Autodesk Inventor part; units mm, degrees
ref_plane "РабПлоскость1" through (25, 2, 0) normal (1, 0, 0) x (0, 0, -1)
ref_plane "РабПлоскость2" through (2, 12.5, 0) normal (0, -1, 0) x (1, 0, 0)
ref_plane "РабПлоскость3" through (25, 25, 5.2) normal (1, 0, 0) x (0, 0, -1)
sketch "Эскиз1" plane through (0, 0, 0) normal (0, 0, 1) x (1, 0, 0)
  line L0 (0, 0) -> (50, 0)
  line L1 (50, 0) -> (50, 25)
  line L2 (50, 25) -> (0, 25)
  line L3 (0, 25) -> (0, 0)
  dimension "d0" = 50
  dimension "d1" = 25
extrude "Выдавливание1" add sketch "Эскиз1" along normal blind 5.2
shell "Оболочка1" thickness 2 removed faces 1 at (16.6667, 16.6667, 0)
sketch "Эскиз2" plane through (0, 0, 5.2) normal (0, 0, 1) x (1, 0, 0)
  line L0 (50, 25) -> (0, 25)
  line L1 (25, 25) -> (25, 0)
  line L2 (0, 0) -> (50, 0)
  line L3 (25, 12.5) -> (12, 12.5)
  line L4 (0, 25) -> (0, 0)
  circle A0 centre (12, 12.5) radius 8.1
  circle A1 centre (38, 12.5) radius 8.1
  line L5 (25, 25) -> (25, 20)
  line L6 (21.75, 20) -> (28.25, 20) construction
  line L7 (21.75, 18) -> (28.25, 18)
  line L8 (28.25, 22) -> (21.75, 22)
  arc A2 (21.75, 22) -> (21.75, 18) centre (21.75, 20) ccw
  arc A3 (28.25, 18) -> (28.25, 22) centre (28.25, 20) ccw
  point P0 (25, 18)
  point P1 (25, 22)
  dimension "d5" = 13
  dimension "d6" = 16.2
  dimension "d9" = 5
  dimension "d10" = 3.25
  dimension "d11" = 4
extrude "Выдавливание2" cut sketch "Эскиз2" against normal through all contours L8 A3 L7 L1 | L1 L7 A2 L8 | A0 | A1
sketch "Эскиз5" plane through (48, 23, 3.2) normal (0, 0, -1) x (-1, 0, 0)
  line L0 (0, 0) -> (1.05, 0)
  line L1 (0, 0) -> (46, 0)
  line L2 (1.05, 0) -> (1.05, -1.05)
  circle A0 centre (1.05, -1.05) radius 1.05
  line L3 (2.1, -2.1) -> (0, -2.1)
  line L4 (0, -2.1) -> (0, 0)
  line L5 (0, 0) -> (2.1, 0)
  line L6 (2.1, 0) -> (2.1, -2.1)
  line L7 (2.1, -2.1) -> (0, 0) construction
  line L8 (0, -2.1) -> (2.1, 0) construction
  point P0 (48, -23)
  point P1 (1.05, -2.1)
  point P2 (2.1, -1.05)
  dimension "d17" = 1.05
  dimension "d18" = 1.05
extrude "Выдавливание4" add sketch "Эскиз5" along normal blind 1 contours L0 A0 L4 | L1 L6 A0 | A0 | A0 L3 L4
ref_plane "РабПлоскость1" through (25, 2, 0) normal (1, 0, 0) x (0, 0, -1)
ref_plane "РабПлоскость2" through (2, 12.5, 0) normal (0, -1, 0) x (1, 0, 0)
mirror "Зеркальное отражение1" about plane through (2, 12.5, 0) normal (0, -1, 0) of "Выдавливание4"
mirror "Зеркальное отражение2" about plane through (25, 2, 0) normal (1, 0, 0) of "Выдавливание4", "Зеркальное отражение1"
sketch "Эскиз10" plane through (0, 0, 0) normal (0, -1, 0) x (1, 0, 0)
  line L0 (0, 0) -> (50, 0)
  line L1 (50, 0) -> (42, 0)
  line L2 (42, 0) -> (42, -8)
  line L3 (42, -8) -> (50, -8)
  line L4 (50, -8) -> (50, 0)
  dimension "d39" = 8
  dimension "d40" = 8
extrude "Выдавливание8" add sketch "Эскиз10" against normal up to surface (2 mm away)
sketch "Эскиз11" plane through (48, 2, 0) normal (0, 1, 0) x (1, 0, 0)
  line L0 (-6, 0) -> (-6, 8)
  line L1 (-6, 4) -> (2, 4)
  line L2 (2, 0) -> (2, 8)
  line L3 (-6, 8) -> (-6, 0)
  point P0 (-48, 0)
  point P1 (-2, 4)
hole "Отверстие2" at (46, 2, -4) direction (0, -1, 0) diameter 3.2 end through all countersink diameter 6 countersink angle 90
ref_plane "РабПлоскость3" through (25, 25, 5.2) normal (1, 0, 0) x (0, 0, -1)
mirror "Зеркальное отражение4" about plane through (25, 25, 5.2) normal (1, 0, 0) of "Отверстие2", "Выдавливание8"
fillet "Сопряжение2" radius 4 6 edges at (42, 1, -8) (50, 1, -8) (8, 1, -8) (0, 1, -8) (8, 1, 0) (42, 1, 0)
sketch "Эскиз12" plane through (0, 0, 5.2) normal (0, -1, 0) x (1, 0, 0)
  circle A0 centre (46, -9.2) radius 1.6
  circle A1 centre (4, -9.2) radius 1.6
  arc A2 (0, -9.2) -> (8, -9.2) centre (4, -9.2) ccw
  arc A3 (12, -5.2) -> (8, -9.2) centre (12, -9.2) ccw
  line L0 (12, -5.2) -> (38, -5.2)
  arc A4 (42, -9.2) -> (38, -5.2) centre (38, -9.2) ccw
  arc A5 (42, -9.2) -> (50, -9.2) centre (46, -9.2) ccw
  line L1 (50, -9.2) -> (50, 0)
  line L2 (0, 0) -> (50, 0)
  line L3 (0, -9.2) -> (0, 0)
  point P0 (0, -5.2)
extrude "Выдавливание9" add sketch "Эскиз12" along normal blind 1
properties part number "Крепление ультрасоника"
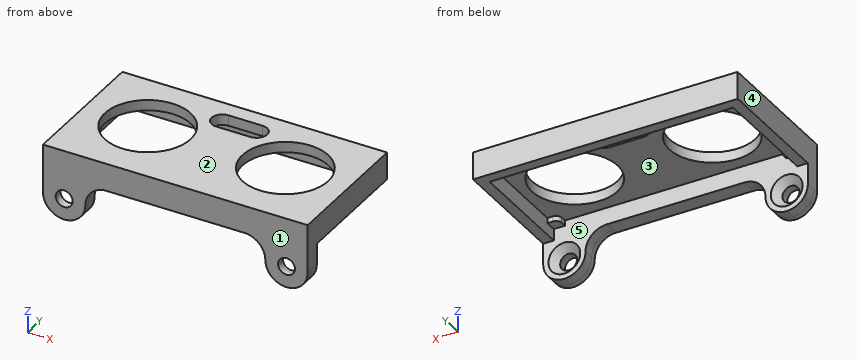
Can you work these out from the model? Positions are in its coordinate system, mm. Face numbers are marked on the shaded views. A direction names the side the tool comes from. Give positions to 0.01 mm unless a question says otherwise; leave off trailing zeros. Order: outer loops, then holes, each group sorted by start corner. A loop starts at its lowest first (then second) coordinate and runs counter-clockwise, first axis right, second up. Notation, with made-up numbers: M 25,-32.5 L 62,-32.5 A24 cw 62,-8.5 Z; hole C 22,-16.5 d11. An arc over 180 degrees is marked long. One line per item, written item: value.
Item 1: If we mould it in two halves opening along Y, with no side actions, what happens to the marked faces 1, 2 and 3? For each: pulls with the +Y half, pulls with the -Y half, needs draft (parallel to the pull), parting line crosses it, or undercut.
Verdict:
face 1: pulls with the -Y half
face 2: needs draft
face 3: undercut
Item 2: If we section it at D-D on y = 2.5: Write out the boundary of the cut face in (x, z).
Verdict:
outline: M 0,0 L 2,0 L 2,2.2 L 4.1,2.2 L 4.1,3.2 L 45.9,3.2 L 45.9,2.2 L 48,2.2 L 48,0 L 50,0 L 50,5.2 L 0,5.2 Z
Item 3: If we section it at B-B on x = 31: Write out the boundary of the cut face in (y, z).
Verdict:
outline: M -1,0 L 2,0 L 2,3.2 L 8.42,3.2 L 8.42,5.2 L -1,5.2 Z; M 16.58,3.2 L 23,3.2 L 23,0 L 25,0 L 25,5.2 L 16.58,5.2 Z
Item 4: If we section it at A-A on y = 12.5: Write out the boundary of the cut face in (x, z), and give its area (3 significant figures).
Verdict:
outline: M 0,0 L 2,0 L 2,3.2 L 3.9,3.2 L 3.9,5.2 L 0,5.2 Z; M 20.1,3.2 L 29.9,3.2 L 29.9,5.2 L 20.1,5.2 Z; M 46.1,3.2 L 48,3.2 L 48,0 L 50,0 L 50,5.2 L 46.1,5.2 Z
area: 48.0 mm2
Item 5: Please list where these lines run through material, in increasing order: line 1 (X direction, y = -0.3, z = -4); line 2 (Y direction, x = 38, z = 4.3); line 3 (Z direction, x = 46, y = 0.35).
Verdict:
line 1: 0 to 2.4, 5.6 to 8, 42 to 44.4, 47.6 to 50
line 2: -1 to 4.4, 20.6 to 25
line 3: -8 to -5.6, -2.4 to 5.2
Item 6: If we section it at C-C on z = 4.25: Write out the boundary of the cut face in (x, y).
Verdict:
outline: M 0,-1 L 50,-1 L 50,25 L 0,25 Z; hole C 12,12.5 d16.2; hole M 21.75,18 L 28.25,18 A2 ccw 28.25,22 L 21.75,22 A2 ccw Z; hole C 38,12.5 d16.2
Item 7: For the marked faces 4 and 5, which set-ups out of +Z, -Z, +X, -X, +Y, -Y let a thin tool reach every point of the face, with its end or its side?
Verdict:
face 4: +Z, -Z, -X, +Y, -Y
face 5: -Z
Item 8: For pin 1 (1 mm diameter, centred on x = 22.5, y = 18, fed in from -Z); pin 2 (3 mm diameter, centred on x = 4, z = -4, fed in from -Y); pin 3 (1.7 mm diameter, centred on x = 3.5, y = 22, fed in from -Z), each with a flat end and sliding along its axis, tell me the tip position at first contact or that it passes through.
Verdict:
pin 1: z = 3.2
pin 2: through
pin 3: z = 2.2
